For this review, take the finished solid that the model builds, in its own axes (mm). Face numbers are marked on the shaded views. A direction names the side the tool comes from. Coordinates: 2 decimals unless noted, no trailing zeros. Loops run counter-clockwise (first coordinate to the right, second up) from the corner with the lowest first, then second, coordinate; pieces in that order, holes last. Notation, with made-up numbers: M -13.5,31 L 9.5,31 A24 cw 9.5,51 Z; hole C 85,39.5 d5. An arc over 180 degrees is marked long. Write item = value, one per line.
from build123d import *

# Parameters (mm, degrees)
F0_W     = 5
F0_H     = 5
F0_W_2   = 3
F0_H_2   = 30
F1_DEPTH = 16
F2_SIZE  = 4.99999
F3_SIZE  = 4.99999
F4_R     = 5
F5_R     = 2.99999


# Not quite as in the source:
# - a fillet or chamfer is up to 0.001 mm smaller than in the source, because OpenCascade refuses the exact size


with BuildPart() as f1:
    # F0 (on Top) → F1 (new body)
    with BuildSketch(Plane.XY):
        with Locations((-37.7777791023, 2.5)):
            Rectangle(F0_W, F0_H)
        Polygon((-35.2777791023, -4), (-35.2777791023, 0), (-40.2777791023, 0), (-40.2777791023, -40), (-35.2777791023, -40), align=None)
        Polygon((2.7222208977, 0), (-35.2777791023, 0), (-35.2777791023, -4), (5.7222208977, -4), (5.7222208977, 0), align=None)
        with Locations((4.2222208977, 15)):
            Rectangle(F0_W_2, F0_H_2)
    extrude(amount=F1_DEPTH)

    # F2 (size 5 in the source; OpenCascade refuses exactly that, so slightly less here)
    f2_edges = [f1.edges().sort_by_distance(p)[0] for p in [
        (-35.277779, 5, 8),
    ]]
    chamfer(f2_edges, length=F2_SIZE)

    # F3 (size 5 in the source; OpenCascade refuses exactly that, so slightly less here)
    f3_edges = [f1.edges().sort_by_distance(p)[0] for p in [
        (-35.277779, -40, 8),
    ]]
    chamfer(f3_edges, length=F3_SIZE)

    # F4
    f4_edges = [f1.edges().sort_by_distance(p)[0] for p in [
        (2.722221, 0, 8),
    ]]
    fillet(f4_edges, radius=F4_R)

    # F5 (radius 3 in the source; OpenCascade refuses exactly that, so slightly less here)
    f5_edges = [f1.edges().sort_by_distance(p)[0] for p in [
        (5.722221, -4, 8),
        (5.722221, 30, 8),
    ]]
    fillet(f5_edges, radius=F5_R)


solid = f1.part
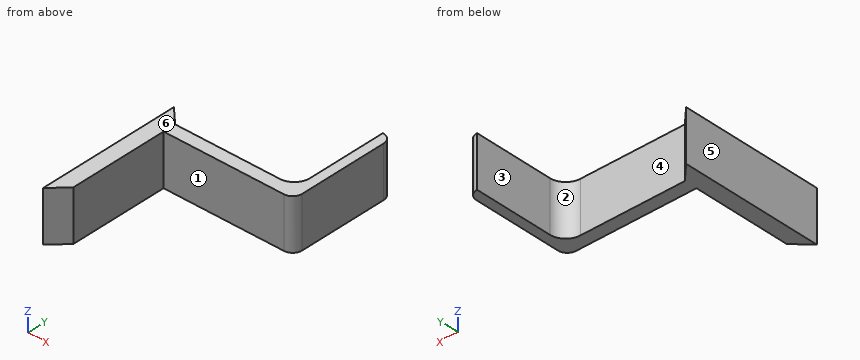
Q1. Add section C-C (x = -27.5). Write out the cut boundary in (y, z), and give its area (3 significant figures).
Solved:
outline = M -4,0 L 0,0 L 0,16 L -4,16 Z
area = 64.0 mm²
Q2. Draft analysis for pull direction X (two halves, no side actions). For the marked faces 4, 5 and 6, state which applies: +X half, -X half, draft (parallel to the pull), parting line (faces both ways), or undercut.
Solved:
face_4 = undercut
face_5 = -X half
face_6 = draft
Q3. Add section B-B (y = 3.5). Write out the cut boundary in (x, z).
Solved:
outline = M -40.28,0 L -38.78,0 L -38.78,16 L -40.28,16 Z; M 2.49,0 L 5.72,0 L 5.72,16 L 2.49,16 Z
Q4. Add section D-D (y = -29.5). Write out the cut boundary in (x, z), and give its area (3 significant figures).
Solved:
outline = M -40.28,0 L -35.28,0 L -35.28,16 L -40.28,16 Z
area = 80.0 mm²
Q5. Machinability: for the marked faces 1, 2 and 3, which of the approach directions +Z, -Z, +X, -X, +Y, -Y give a long, thin tool a straight path to every point of the face, cutting with its end or side? Answer none if there is none.
Solved:
face_1 = +Z, -Z, +X, -Y
face_2 = +Z, -Z, +Y
face_3 = +Z, -Z, -X, +Y
Q6. For pin 1 Ø8 at (x, z) = (-25.5, 6) entering from +Y; pin 2 Ø2 at (x, z) = (-21.5, 12.5) entering from -Y; pin 3 Ø1.5 at (y, z) = (-4.5, 7) entering from +X, all flat-tipped, find the tip position at first contact; note any pin that passes through.
Solved:
pin_1 = 0
pin_2 = -4
pin_3 = 3.92
Q7. For line 1 along Y through (x, z) = (-30.5, 2.5); line 2 along X through (y, z) = (-26.5, 7.5); line 3 along X through (y, z) = (15.5, 2.75), list the stretches that pass through material, from the lowest coordinate up.
Solved:
line_1 = -4 to 0
line_2 = -40.28 to -35.28
line_3 = 2.72 to 5.72
